The model under review builds one solid part; all positions refer to its coordinate system, in mm. A direction names the side the tool comes from. Round coordinates to 2 decimals unless told otherwise and drop trailing zeros. Loops run counter-clockwise (first coordinate to the right, second up) from the corner with the lowest first, then second, coordinate; pieces in that order, holes last. Notation, with made-up numbers: M -7.5,9.25 L 30.5,9.25 A23 ccw 30.5,33.25 Z; hole C -24,0.25 d11. An arc over 180 degrees is marked long. Return JSON: item names as keys, results as strings. Group by question number.
Q1. Draft analysis for pull direction Z (two halves, no side actions). For faces 1 (the face through (6.466, 1.479, 2.681)), 2 (the face through (40, 0, -62)), 3 (the face through (48, 1, -113)), 4 (the face through (-165.15, 1.48, -52.99)), state which applies: pulls with the +Z half, pulls with the -Z half, needs draft (parallel to the pull), parting line crosses it, or undercut.
Q2. Consider section B-B (x = 0). State the section outline as (y, z) points, and give its area (3 significant figures).
Q3. Consider section A-A (x = 89.5). State the section outline as (y, z) points, and give its area (3 significant figures).
Q4. Consider section C-C (y = 1.95). Count the separate pieces of the cut face and the enclosed holes in it, and give its area (3 significant figures).
Q5. To check wall thickness, follow line 1 along X through (y, z) = (1.45, -200); line 2 along X through (y, z) = (2.25, 0); line 3 along Z through (x, y) = (-16, 1.7). State the ranges of each line that lie inside material, in increasing order.
Q6. For faces 5 (the face through (48, 1, -178)), 6 (the face through (164.99, 1.48, -213.15)), list the 3-axis set-ups (+Z, -Z, +X, -X, +Y, -Y) from which the entire face can be reached by the end or side of a thin tool; tool diameter is ignored.
Q7. Consider section D-D (z = -151). State the section outline as (x, y) points, and give its area (3 significant figures).
Q8. Clearance check with flat-ended pins moving along their axes: pin 1 Ø3.5 at (x, z) = (16, -208) entering from +Y; pin 2 Ø1.5 at (x, y) = (-74, 1) entering from -Z. State where each tip first meets the part, or that it passes through.
from build123d import *

# Parameters (mm, degrees)
SKETCH1_R               = 7
SKETCH1_R_2             = 2.1
BOSS_EXTRUDE1_DEPTH     = 3
SKETCH2_W               = 336
SKETCH2_H               = 4
CUT_EXTRUDE1_DEPTH      = 1
CUT_EXTRUDE1_DEPTH_BACK = 4


with BuildPart() as part:
    # Sketch1 → Boss-Extrude1 (new body)
    with BuildSketch(Plane(origin=(0, 0, 0), x_dir=(1, 0, 0), z_dir=(0, 1, 0))):
        with BuildLine():
            Line((-23, 216), (158, 216))
            ThreePointArc((158, 216), (165.071067812, 213.071067812), (168, 206))
            Line((168, 206), (168, -43))
            Line((168, -43), (-168, -43))
            Line((-168, -43), (-168, 46))
            ThreePointArc((-168, 46), (-165.071067812, 53.071067812), (-158, 56))
            Line((-158, 56), (-27, 56))
            ThreePointArc((-27, 56), (-24.171572875, 57.171572875), (-23, 60))
            Line((-23, 60), (-23, 216))
        make_face()
        Circle(SKETCH1_R, mode=Mode.SUBTRACT)
        with Locations((16, 8)):
            Circle(SKETCH1_R_2, mode=Mode.SUBTRACT)
        with Locations((16, -8)):
            Circle(SKETCH1_R_2, mode=Mode.SUBTRACT)
        with Locations((16, 208)):
            Circle(SKETCH1_R_2, mode=Mode.SUBTRACT)
        with Locations((16, 184)):
            Circle(SKETCH1_R_2, mode=Mode.SUBTRACT)
        with Locations((16, 200)):
            Circle(SKETCH1_R_2, mode=Mode.SUBTRACT)
        with Locations((-16, 184)):
            Circle(SKETCH1_R_2, mode=Mode.SUBTRACT)
        with Locations((-16, 200)):
            Circle(SKETCH1_R_2, mode=Mode.SUBTRACT)
        with Locations((-16, 208)):
            Circle(SKETCH1_R_2, mode=Mode.SUBTRACT)
        with Locations((-16, -8)):
            Circle(SKETCH1_R_2, mode=Mode.SUBTRACT)
        with Locations((-16, 8)):
            Circle(SKETCH1_R_2, mode=Mode.SUBTRACT)
        with BuildLine():
            Line((-103.5, -27.189984024), (-103.5, 24))
            ThreePointArc((-103.5, 24), (-104.671572875, 26.828427125), (-107.5, 28))
            Line((-107.5, 28), (-126.109686491, 28))
            ThreePointArc((-126.109686491, 28), (-128.938113615, 29.171572875), (-130.109686491, 32))
            Line((-130.109686491, 32), (-130.109686491, 40))
            ThreePointArc((-130.109686491, 40), (-128.938113615, 42.828427125), (-126.109686491, 44))
            Line((-126.109686491, 44), (-64.890313509, 44))
            ThreePointArc((-64.890313509, 44), (-62.061886385, 42.828427125), (-60.890313509, 40))
            Line((-60.890313509, 40), (-60.890313509, 32))
            ThreePointArc((-60.890313509, 32), (-62.061886385, 29.171572875), (-64.890313509, 28))
            Line((-64.890313509, 28), (-83.5, 28))
            ThreePointArc((-83.5, 28), (-86.328427125, 26.828427125), (-87.5, 24))
            Line((-87.5, 24), (-87.5, -27.189984024))
            ThreePointArc((-87.5, -27.189984024), (-88.671572875, -30.018411149), (-91.5, -31.189984024))
            Line((-91.5, -31.189984024), (-99.5, -31.189984024))
            ThreePointArc((-99.5, -31.189984024), (-102.328427125, -30.018411149), (-103.5, -27.189984024))
        make_face(mode=Mode.SUBTRACT)
        with BuildLine():
            Line((60, 60), (132, 60))
            ThreePointArc((132, 60), (144, 48), (132, 36))
            Line((132, 36), (60, 36))
            ThreePointArc((60, 36), (48, 48), (60, 60))
        make_face(mode=Mode.SUBTRACT)
        with BuildLine():
            Line((60, 125), (132, 125))
            ThreePointArc((132, 125), (144, 113), (132, 101))
            Line((132, 101), (60, 101))
            ThreePointArc((60, 101), (48, 113), (60, 125))
        make_face(mode=Mode.SUBTRACT)
        with BuildLine():
            Line((60, 190), (132, 190))
            ThreePointArc((132, 190), (144, 178), (132, 166))
            Line((132, 166), (60, 166))
            ThreePointArc((60, 166), (48, 178), (60, 190))
        make_face(mode=Mode.SUBTRACT)
    extrude(amount=BOSS_EXTRUDE1_DEPTH)

    # Sketch2 → Cut-Extrude1 (cut, two sides)
    with BuildSketch(Plane(origin=(0, 3, 0), x_dir=(1, 0, 0), z_dir=(0, 1, 0))) as cut_extrude1_sk:
        with Locations((0, -41)):
            Rectangle(SKETCH2_W, SKETCH2_H)
    extrude(amount=CUT_EXTRUDE1_DEPTH, mode=Mode.SUBTRACT)
    extrude(cut_extrude1_sk.sketch, amount=-CUT_EXTRUDE1_DEPTH_BACK, mode=Mode.SUBTRACT)


solid = part.part
Values:
{
 "1": {"face 1": "undercut", "face 2": "needs draft", "face 3": "undercut", "face 4": "pulls with the -Z half"},
 "2": {"outline": "M 0,-216 L 3,-216 L 3,-7 L 0,-7 Z; M 0,7 L 3,7 L 3,39 L 0,39 Z", "area": "723 mm2"},
 "3": {"outline": "M 0,-216 L 3,-216 L 3,-190 L 0,-190 Z; M 0,-166 L 3,-166 L 3,-125 L 0,-125 Z; M 0,-101 L 3,-101 L 3,-60 L 0,-60 Z; M 0,-36 L 3,-36 L 3,39 L 0,39 Z", "area": "549 mm2"},
 "4": {"separate pieces": "1", "enclosed holes": "15", "area": "53,600 mm2"},
 "5": {"line 1": "x = -23 to -18.1, -13.9 to 13.9, 18.1 to 168", "line 2": "x = -168 to -103.5, -87.5 to -7, 7 to 168", "line 3": "z = -216 to -210.1, -205.9 to -202.1, -197.9 to -186.1, -181.9 to -10.1, -5.9 to 5.9, 10.1 to 39"},
 "6": {"face 5": "+Y, -Y", "face 6": "-Z, +X, +Y, -Y"},
 "7": {"outline": "M -23,0 L 168,0 L 168,3 L -23,3 Z", "area": "573 mm2"},
 "8": {"pin 1": "passes through", "pin 2": "stops at z = -56"}
}
